Design review of the part shown in the three views and the two pictorial views. Dimensions are in mm from the part's minimum x, y and z. Give positions to 0.01 mm unless a question says otherwise; leave off trailing zeros. Write each loop counter-clockwise with the first axis right and the second up, starting at its lowest first coordinate (ties: lowest second). Pieces come first, ordered by that corner, then holes. Notation, with made-up numbers: (64.25, -16.75) -> (80.25, -16.75) arc R37 ccw to (80.25, 22.25) -> close; hole circle Ø4 at (-15, -10.75). An arc over 180 degrees is marked (long way). Return JSON: item names as keys, results as strings. Group by question number.
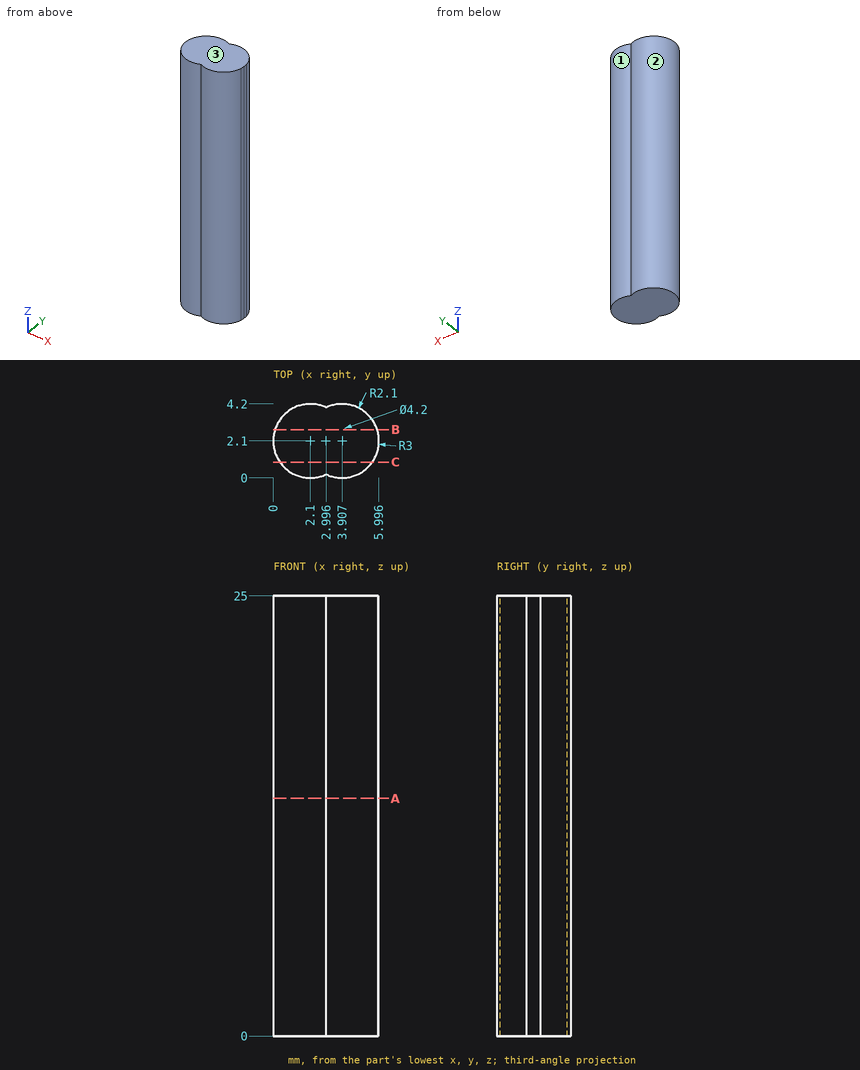
Q1. Mouldability with a two-part tool opening along X and no side actions: class the marked faces 1, 2 and 3 as +X half, -X half, draft (parallel to the pull), parting line (faces both ways), or undercut.
Q2. Take a section at A-A, the plane z = 13.5. Give the boundary of the cut face in (x, y) (1 decimal), plus the area to 3 significant figures.
Q3. Insertion check: pin 1 (1.5 mm diameter, centred on x = 4.5, y = 3.5, fed in from -Z); pin 2 (1 mm diameter, centred on x = 5.5, z = 16, fed in from -Y); pin 3 (2 mm diameter, centred on x = 1, z = 21.5, fed in from +Y). Each pin has a flat end and moves straight along its axis. Give the tip position at first contact, or say it passes through.
Q4. Take a section at C-C, the plane y = 0.9. Give the boundary of the cut face in (x, z).
Q5. For L1, parallel to Y at x = 3.8, z = 10.25; L2, parallel to X at y = 1.35, z = 22.5; L3, parallel to Y at x = 4.6, z = 20.75, list the stretches that pass through material, from the lowest coordinate up. Write a range as from..to.
Q6. Take a section at B-B, the plane y = 2.75. Give the boundary of the cut face in (x, z).
Final values:
{
 "1": {"face 1": "undercut", "face 2": "undercut", "face 3": "draft"},
 "2": {"outline": "(3, 0.2) arc R2.1 ccw to (6, 1.7) arc R3 ccw to (6, 2.5) arc R2.1 ccw to (3, 4) arc R2.1 ccw (long way) to start", "area": "21.2 mm²"},
 "3": {"pin 1": "stops at z = 0", "pin 2": "stops at y = 0.31", "pin 3": "stops at y = 4.2"},
 "4": {"outline": "(0.38, 0) -> (5.63, 0) -> (5.63, 25) -> (0.38, 25) -> close"},
 "5": {"L1": "y = 0..4.2", "L2": "x = 0.14..5.87", "L3": "y = 0.12..4.08"},
 "6": {"outline": "(0.1, 0) -> (5.9, 0) -> (5.9, 25) -> (0.1, 25) -> close"}
}
